```python
from build123d import *

# Parameters (mm, degrees)
F1_DEPTH = 76.2


with BuildPart() as f1:
    # F0 (on Top) → F1 (new body)
    with BuildSketch(Plane.XY):
        Polygon((0, 50.8), (0, 25.4), (71.842049, 0), (71.842049, 76.2), align=None)
        Polygon((-76.2, 76.2), (-76.2, 0), (0, 0), (0, 25.4), (0, 50.8), (0, 76.2), align=None)
    extrude(amount=-F1_DEPTH)


solid = f1.part
```
Work out the finished part from the listing and answer in its coordinate system (mm). A direction names the side the tool comes from. Round coordinates to 2 decimals unless told otherwise and drop trailing zeros. Write each loop counter-clockwise with the first axis right and the second up, starting at its lowest first coordinate (ties: lowest second). Pieces come first, ordered by that corner, then holes. Notation, with made-up numbers: (85.5, 85) - (94.5, 85) arc R26 cw to (94.5, 103) - close; hole circle Ø7 at (23.25, -3). An arc over 180 degrees is marked (long way). Return JSON: item names as keys, results as strings. Group by question number.
Q1. Find the intervals of material crossed by L1, parallel to Y at x = 51, z = -39; L2, parallel to Y at x = 18, z = -33, in increasing order.
Q2. The part is cut by section D-D on x = 10.5. Write down the section's boundary in (y, z).
Q3. The part is cut by section B-B on y = 5. Write down the section's boundary in (x, z).
Q4. For faces 5 (the flat face through (0, 63, -38)), 6 (the flat face through (0, 13, -38)), 7 (the flat face through (-3, 39, -76.2)), determine the directions among +Z, -Z, +X, -X, +Y, -Y from which every point of the face is accessible in a straight line to the end or side of a thin tool.
Q5. The part is cut by section C-C on x = 61.5. Write down the section's boundary in (y, z).
Q6. The part is cut by section A-A on z = -52. Write down the section's boundary in (x, y).
Q7. The mould has two halves that part along X. Classify faces 1 (the flat face through (36.424, 63.678, -37.567)), 2 (the flat face through (-39, 0, -38)), 3 (the flat face through (-76.2, 39, -38)), 4 (the flat face through (71.842, 38, -38)): released by +X, released by -X, zero draft, split by the parting line, or undercut.
Q8. Each of these flat-tipped pins is pushed along its axis until it touches: pin 1 Ø2 at (x, z) = (-50.5, -49) entering from -Y; pin 2 Ø5 at (x, z) = (24.5, -44.5) entering from -Y. Where does it stop, or does it pass through?
Solved:
{
 "1": {"L1": "7.37 to 68.83", "L2": "19.04 to 57.16"},
 "2": {"outline": "(21.69, -76.2) - (54.51, -76.2) - (54.51, 0) - (21.69, 0) - close"},
 "3": {"outline": "(-76.2, -76.2) - (0, -76.2) - (0, 0) - (-76.2, 0) - close; (57.7, -76.2) - (71.84, -76.2) - (71.84, 0) - (57.7, 0) - close"},
 "4": {"face 5": "+Z, -Z, +Y", "face 6": "+Z, -Z, -Y", "face 7": "-Z, +X, -X, +Y, -Y"},
 "5": {"outline": "(3.66, -76.2) - (72.54, -76.2) - (72.54, 0) - (3.66, 0) - close"},
 "6": {"outline": "(-76.2, 0) - (0, 0) - (0, 25.4) - (71.84, 0) - (71.84, 76.2) - (0, 50.8) - (0, 76.2) - (-76.2, 76.2) - close"},
 "7": {"face 1": "undercut", "face 2": "zero draft", "face 3": "released by -X", "face 4": "released by +X"},
 "8": {"pin 1": "y = 0", "pin 2": "y = 15.85"}
}
